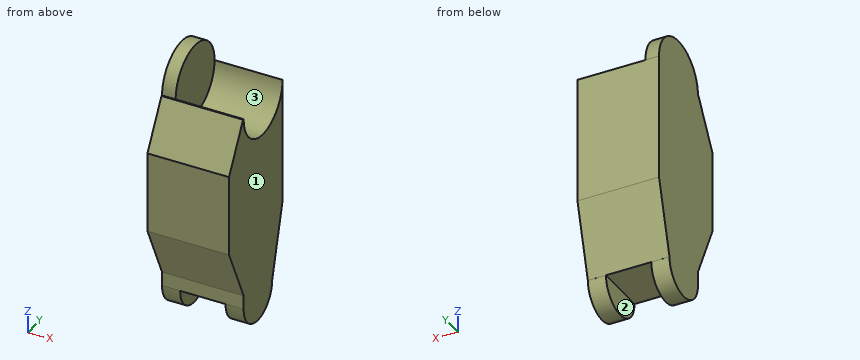
from build123d import *

# Parameters (mm, degrees)
F1_DEPTH     = 19.05
F2_DEPTH     = 114.3
F3_W         = 114.3
F3_H         = 101.6
F4_DEPTH     = 177.8
F5_T1_DEPTH  = 641.9538230647
F6_R         = 37.1475
F7_DEPTH     = 25.4
F8_R         = 37.1475
F9_DEPTH     = 25.4
F10_W        = 114.3
F10_H        = 266.7
F11_DEPTH    = 38.1
F12_T4_DEPTH = 574.9754388191
F13_T1_DEPTH = 442.85989084


# Not quite as in the source:
# - a fillet or chamfer that OpenCascade refuses, or shapes differently, is made with other operations: its cross-section is extruded or revolved along the edge and cut away or added


with BuildPart() as f1:
    # F0 (on Right) → F1 (new body)
    with BuildSketch(Plane.YZ):
        with BuildLine():
            Line((-50.8, 0), (50.8, 0))
            ThreePointArc((50.8, 0), (0, 50.8), (-50.8, 0))
        make_face()
        with BuildLine():
            Line((50.8, -101.6), (50.8, 0))
            ThreePointArc((50.8, 0), (0, -50.8), (-50.8, 0))
            Line((-50.8, 0), (-50.8, -101.6))
            Line((-50.8, -101.6), (50.8, -101.6))
        make_face()
        with BuildLine():
            ThreePointArc((-50.8, 0), (0, -50.8), (50.8, 0))
            Line((50.8, 0), (-50.8, 0))
        make_face()
    extrude(amount=F1_DEPTH)

    # F0 (on Right) → F2 (join)
    with BuildSketch(Plane.YZ):
        with BuildLine():
            Line((50.8, -101.6), (50.8, 0))
            ThreePointArc((50.8, 0), (0, -50.8), (-50.8, 0))
            Line((-50.8, 0), (-50.8, -101.6))
            Line((-50.8, -101.6), (50.8, -101.6))
        make_face()
    extrude(amount=F2_DEPTH)

    # F3 (on face) → F4 (join)
    with BuildSketch(Plane(origin=(0, 0, -101.6), x_dir=(1, 0, 0), z_dir=(0, 0, -1))):
        with Locations((57.15, 0)):
            Rectangle(F3_W, F3_H)
    extrude(amount=F4_DEPTH)

    # F5: chamfer of 101.6 x 27.223637951 on 1 edges, made by hand

    # F5_s2 → F5_t1 (cut)
    with BuildSketch(Plane.YZ.offset(-263.8269115324)):
        Polygon((23.576362049, -279.4), (50.8, -177.8), (50.8, -279.4), align=None)
    extrude(amount=F5_T1_DEPTH, mode=Mode.SUBTRACT)

    # F6 (on face) → F7 (join)
    with BuildSketch(Plane(origin=(0, 0, 0), x_dir=(0, -1, 0), z_dir=(-1, 0, 0))):
        with Locations((13.6118189755, -279.4)):
            Circle(F6_R)
    extrude(amount=-F7_DEPTH)

    # F8 (on face) → F9 (join)
    with BuildSketch(Plane.YZ.offset(114.3)):
        with Locations((-13.6118189755, -279.4)):
            Circle(F8_R)
    extrude(amount=-F9_DEPTH)

    # F10 (on face) → F11 (join)
    with BuildSketch(Plane.XZ.offset(50.8)):
        with Locations((57.15, -133.35)):
            Rectangle(F10_W, F10_H)
    extrude(amount=F11_DEPTH)

    # F12: chamfer of 88.9 x 41.45475081 on 1 edges, made by hand


with BuildPart() as f12_tool2:
    # F12_s3 → F12_t4 (new body)
    with BuildSketch(Plane.YZ.offset(-230.3377194096)):
        Polygon((-88.9, -177.8), (-47.44524919, -266.7), (-88.9, -266.7), align=None)
    extrude(amount=F12_T4_DEPTH)

    split(bisect_by=Plane.XZ.offset(50.8), keep=Keep.TOP)


with BuildPart() as f1_1:
    add(f1.part)

    # F12_t1: cut F12_tool2
    add(f12_tool2.part, mode=Mode.SUBTRACT)

    # F13: chamfer of 63.5 x 36.6617420935 on 1 edges, made by hand

    # F13_s2 → F13_t1 (cut)
    with BuildSketch(Plane.YZ.offset(-164.27994542)):
        Polygon((-88.9, -63.5), (-52.2382579065, 0), (-88.9, 0), align=None)
    extrude(amount=F13_T1_DEPTH, mode=Mode.SUBTRACT)


solid = f1_1.part
Geometry: final body of the model. Coordinates: model frame, mm. Face numbers are marked on the shaded views. A direction names the side the tool comes from. Round coordinates to 2 decimals unless told otherwise and drop trailing zeros. Order: outer loops, then holes, each group sorted by start corner. A loop starts at its lowest first (then second) coordinate and runs counter-clockwise, first axis right, second up.
Q1. Material intervals for probe 1 along X at (y, z) = (-1.5, -285); probe 2 along Y at (x, z) = (105, -42); probe 3 along Z at (x, y) = (40, 7), sorted ascending.
Result sheet:
probe 1: x = 0 to 25.4, 88.9 to 114.3
probe 2: y = -76.49 to -28.58, 28.58 to 50.8
probe 3: z = -279.4 to -50.32
Q2. Section D-D, the plane y = 4. Output: boundary loops of the cut face in (x, z), and give its area (3 significant figures).
Result sheet:
outline: (0, -312.11) - (25.4, -312.11) - (25.4, -279.4) - (88.9, -279.4) - (88.9, -312.11) - (114.3, -312.11) - (114.3, -50.64) - (19.05, -50.64) - (19.05, 50.64) - (0, 50.64) - close
area: 29,700 mm2
Q3. Access query for the marked faces 1, 2 and 3. Directions: +Z, -Z, +X, -X, +Y, -Y. A direction counts if a zero-diameter tool reaches every point of the face in a straight line with its end or side. Return the directions, or none.
Result sheet:
face 1: +Z, -Z, +X, +Y, -Y
face 2: -Z, +Y, -Y
face 3: +Z, +X
Q4. Section C-C, the plane y = 19. Output: boundary loops of the cut face in (x, z).
Result sheet:
outline: (0, -297.19) - (25.4, -297.19) - (25.4, -279.4) - (88.9, -279.4) - (88.9, -297.19) - (114.3, -297.19) - (114.3, -47.11) - (19.05, -47.11) - (19.05, 47.11) - (0, 47.11) - close
Q5. Section B-B, the plane z = -288. Output: boundary loops of the cut face in (x, y), and give its area (3 significant figures).
Result sheet:
outline: (0, -49.75) - (25.4, -49.75) - (25.4, 22.53) - (0, 22.53) - close; (88.9, -49.75) - (114.3, -49.75) - (114.3, 22.53) - (88.9, 22.53) - close
area: 3,670 mm2
Q6. Pin query (flat end, axial travel): pin 1 (8 mm diameter, centred on x = 31, z = -193, fed in from +Y); pin 2 (6 mm diameter, centred on x = 96.5, z = -237, fed in from +Y); pin 3 (4 mm diameter, centred on x = 16, y = -30, fed in from -Z). Return the tip coordinate at first contact, or that it passes through.
Result sheet:
pin 1: stops at y = 47.8
pin 2: stops at y = 35.74
pin 3: stops at z = -313.65
Q7. Section A-A, the plane x = 61. Output: boundary loops of the cut face in (y, z), and give its area (3 significant figures).
Result sheet:
outline: (-88.9, -177.8) - (-50.8, -259.51) - (-50.8, -279.4) - (23.58, -279.4) - (50.8, -177.8) - (50.8, 0) arc R50.8 cw to (-50.8, 0) - (-52.24, 0) - (-88.9, -63.5) - close
area: 30,100 mm2
